Study the drawing (mm; zero at the part's minimum x, y, z) and answer. A direction names the side the tool comes from. Coordinates: 2 decimals unless noted, no trailing zeros. Order: outer loops, then holes, each group sorted by start corner. A loop starts at its lowest first (then second) coordinate and runs counter-clockwise, first axis right, second up. Notation, with made-up numbers: M 54.5,-33 L 60.5,-33 A22 cw 60.5,1 Z; hole C 43,-10.75 d9. An arc over 180 degrees is marked long. Use a Markdown table: item, result. Add a question column.
1) For the marked faces 4 and 5, determine the directions among +Z, -Z, +X, -X, +Y, -Y from which every point of the face is accessible in a straight line to the end or side of a thin tool.
2) The mould has two halves that part along Z. Classify the marked faces 1, 2 and 3: released by +Z, released by -Z, zero draft, split by the parting line, or undercut.
3) Find the intervals of material crossed by probe 1 along X at (y, z) = (2.45, 2.5); probe 2 along X at (y, z) = (0.4, 3.75); probe 3 along Z at (x, y) = (9.45, 2.3), in increasing order. Write a range as [from, to].
4) This flat-tipped pin is pushed along its axis until it touches: pin 1 Ø1.2 at (y, z) = (1.5, 4.5) entering from +X. Where does it stop, or does it pass through?
5) Find section B-B on z = 2. Write down the section's boundary in (x, y).
6) Find section A-A on y = 1.05. Count the separate pieces of the cut face and the enclosed holes in it, plus the area to 3 significant figures.
7) Find section C-C on x = 9.45. Write down the section's boundary in (y, z), plus the area to 3 significant figures.
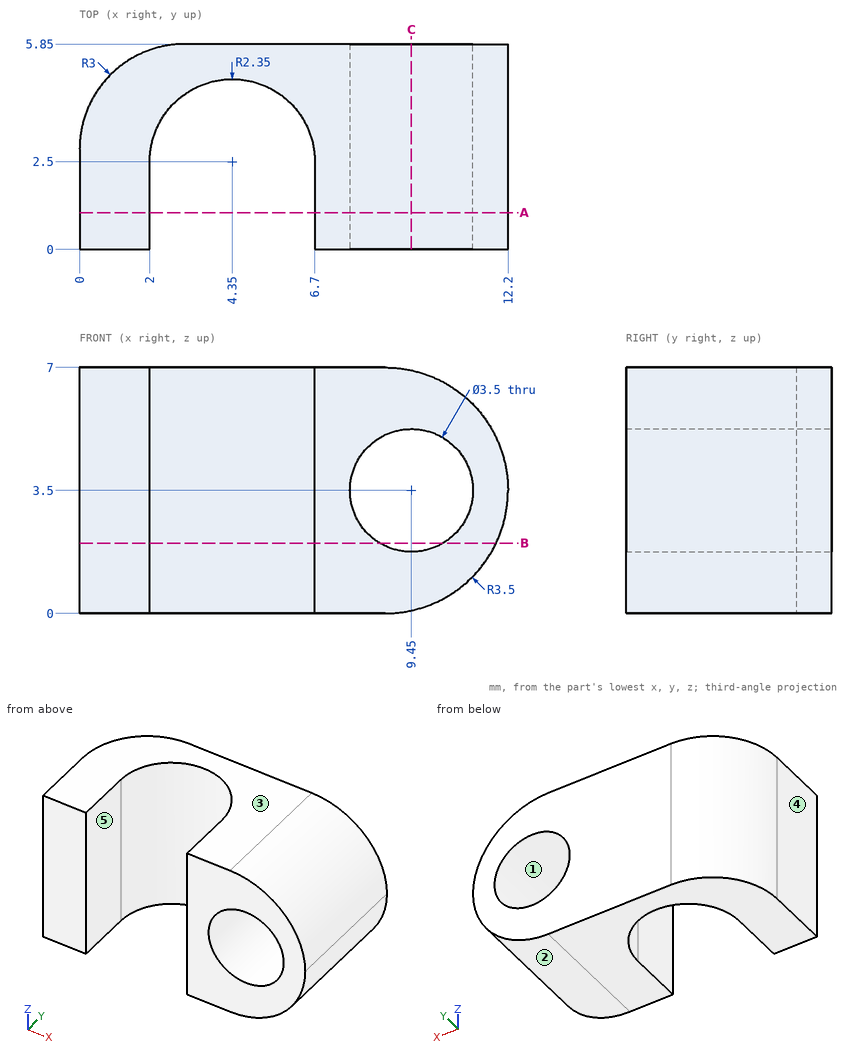
Check result:
| question | item | result |
|---|---|---|
| 1 | face 4 | +Z, -Z, -X, +Y, -Y |
| 1 | face 5 | +Z, -Z, -Y |
| 2 | face 1 | undercut |
| 2 | face 2 | released by -Z |
| 2 | face 3 | released by +Z |
| 3 | probe 1 | x = [0, 2], [6.7, 8.01], [10.89, 12.05] |
| 3 | probe 2 | x = [0, 2], [6.7, 7.72], [11.18, 12.19] |
| 3 | probe 3 | z = [0.08, 1.75], [5.25, 6.92] |
| 4 | pin 1 | stops at x = 12.18 |
| 5 | outline | M 0,0 L 2,0 L 2,2.5 A2.35 cw 6.7,2.5 L 6.7,0 L 8.55,0 L 8.55,5.85 L 3,5.85 A3 ccw 0,2.85 Z; M 10.35,0 L 11.86,0 L 11.86,5.85 L 10.35,5.85 Z |
| 6 | separate pieces | 2 |
| 6 | enclosed holes | 1 |
| 6 | area | 37.6 mm2 |
| 7 | outline | M 0,0.08 L 5.85,0.08 L 5.85,1.75 L 0,1.75 Z; M 0,5.25 L 5.85,5.25 L 5.85,6.92 L 0,6.92 Z |
| 7 | area | 19.5 mm2 |
